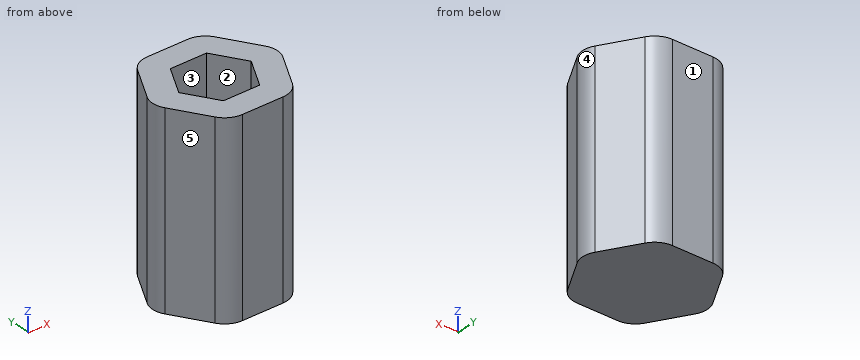
Autodesk Fusion 360 part; units mm, degrees
sketch "Sketch1" plane through (0, 0, 0) normal (0, 0, 1) x (1, 0, 0)
  line L0 (-1.2861, 2.2276) -> (-2.5722, 0)
  line L1 (-2.5722, 0) -> (-1.2861, -2.2276)
  line L2 (-1.2861, -2.2276) -> (1.2861, -2.2276)
  line L3 (1.2861, -2.2276) -> (2.5722, 0)
  line L4 (2.5722, 0) -> (1.2861, 2.2276)
  line L5 (1.2861, 2.2276) -> (-1.2861, 2.2276)
  line L6 (-2.3094, 4) -> (-4.6188, 0)
  line L7 (-4.6188, 0) -> (-2.3094, -4)
  line L8 (-2.3094, -4) -> (2.3094, -4)
  line L9 (2.3094, -4) -> (4.6188, 0)
  line L10 (4.6188, 0) -> (2.3094, 4)
  line L11 (2.3094, 4) -> (-2.3094, 4)
extrude "Extrude1" add sketch "Sketch1" along normal blind 13
extrude "Extrude2" add sketch "Sketch1" along normal blind 1 contours L0 L1 L2 L3 L4 L5
chamfer "Chamfer1" distance 0.5 angle 45 6 edges at (1.9291, -1.1138, 1) (1.9291, 1.1138, 1) (0, 2.2276, 1) (-1.9291, 1.1138, 1) (-1.9291, -1.1138, 1) (0, -2.2276, 1)
fillet "Fillet1" radius 1.5 6 edges at (2.3094, 4, 6.5) (-2.3094, 4, 6.5) (-4.6188, 0, 6.5) (-2.3094, -4, 6.5) (2.3094, -4, 6.5) (4.6188, 0, 6.5)
Can you work these out from the model? Positions are in its coordinate system, mm. Face numbers are marked on the shaded views. A direction names the side the tool comes from. Coordinates: 2 decimals unless noted, no trailing zeros. Write each loop counter-clockwise with the first axis right and the second up, starting at its lowest first coordinate (ties: lowest second). Pieces come first, ordered by that corner, then holes. Notation, with made-up numbers: M 73,37.5 L 103,37.5 A33 cw 103,75.5 Z; hole C 82,34 d4. An arc over 180 degrees is marked long. Use one line per item in the form item = value.
Q1. If we section it at C-C (y = -0.5): Write out the boundary of the cut face in (x, z), then the cut area to 3 significant figures.
Model answer:
outline = M -4.3,0 L 4.3,0 L 4.3,13 L 2.28,13 L 2.28,1.5 L 1.71,1 L -1.71,1 L -2.28,1.5 L -2.28,13 L -4.3,13 Z
area = 57.3 mm^2
Q2. For the marked faces 1 and 2, which set-ups out of +Z, -Z, +X, -X, +Y, -Y let a thin tool reach every point of the face, with its end or its side?
Model answer:
face_1 = +Z, -Z, +X, -X, +Y
face_2 = +Z
Q3. I need wall thicknesses on line 1 along Y through (x, z) = (0.75, 9); line 2 along Z through (x, y) = (-1.75, 0.25); line 3 along Y through (x, z) = (2, 6.5). Which ranges of each line are inside material? Lowest first, please. Write a range as from..to.
Model answer:
line_1 = -4..-2.23, 2.23..4
line_2 = 0..1
line_3 = -3.89..-0.99, 0.99..3.89
Q4. If we section it at A-A (z = 5.5): Write out the boundary of the cut face in (x, y).
Model answer:
outline = M -4.19,-0.75 L -2.74,-3.25 A1.5 ccw -1.44,-4 L 1.44,-4 A1.5 ccw 2.74,-3.25 L 4.19,-0.75 A1.5 ccw 4.19,0.75 L 2.74,3.25 A1.5 ccw 1.44,4 L -1.44,4 A1.5 ccw -2.74,3.25 L -4.19,0.75 A1.5 ccw Z; hole M -2.57,0 L -1.29,-2.23 L 1.29,-2.23 L 2.57,0 L 1.29,2.23 L -1.29,2.23 Z
Q5. If we section it at D-D (x = 3): Write out the boundary of the cut face in (y, z), then the cut area to 3 significant figures.
Model answer:
outline = M -2.8,0 L 2.8,0 L 2.8,13 L -2.8,13 Z
area = 72.9 mm^2
Q6. If we section it at B-B (x = 0.75): Write out the boundary of the cut face in (y, z), then the cut area to 3 significant figures.
Model answer:
outline = M -4,0 L 4,0 L 4,13 L 2.23,13 L 2.23,1.5 L 1.73,1 L -1.73,1 L -2.23,1.5 L -2.23,13 L -4,13 Z
area = 50.8 mm^2
Q7. We'd pull the mould along Y, two halves only. Please class the marked faces 3, 4 and 5: +Y half, -Y half, draft (parallel to the pull), parting line (faces both ways), or undercut.
Model answer:
face_3 = undercut
face_4 = parting line
face_5 = -Y half
Q8. For P1, Ø5, axis at x = 2, z = 2.5, coming from the +Y side; P2, Ø1.7, axis at x = 1, y = -0.5, coming from the +Z side, each with a flat end and sliding along its axis, tell me the tip position at first contact or that it passes through.
Model answer:
P1 = 4
P2 = 1.24
